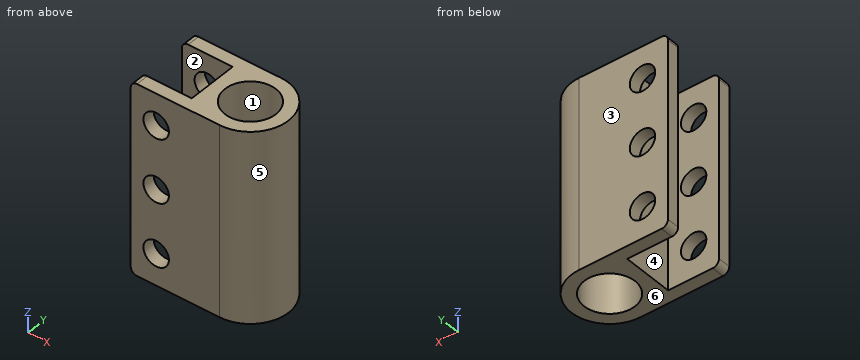
from build123d import *

# Parameters (mm, degrees)
F0_R     = 20
F1_DEPTH = 75
F2_W     = 40
F2_H     = 150
F3_DEPTH = 40
F4_R     = 10
F5_DEPTH = 60
F6_R     = 5
F7_T     = -2


with BuildPart() as f1:
    # F0 (on Top) → F1 (new body, symmetric)
    with BuildSketch(Plane.XY):
        with BuildLine():
            ThreePointArc((30, 0), (21.2132034356, 21.2132034356), (0, 30))
            ThreePointArc((0, 30), (-30, 0), (0, -30))
            ThreePointArc((0, -30), (21.2132034356, -21.2132034356), (30, 0))
        make_face()
        Circle(F0_R, mode=Mode.SUBTRACT)
        with BuildLine():
            Line((0, 30), (-70, 30))
            Line((-70, 30), (-70, -30))
            Line((-70, -30), (0, -30))
            ThreePointArc((0, -30), (-30, 0), (0, 30))
        make_face()
    extrude(amount=F1_DEPTH, both=True)

    # F2 (on face) → F3 (cut)
    with BuildSketch(Plane(origin=(-70, 0, 0), x_dir=(0, -1, 0), z_dir=(-1, 0, 0))):
        Rectangle(F2_W, F2_H)
    extrude(amount=-F3_DEPTH, mode=Mode.SUBTRACT)

    # F4 (on face) → F5 (cut)
    with BuildSketch(Plane.XZ.offset(30)):
        with Locations((-50, 50)):
            Circle(F4_R)
        with Locations((-50, 0)):
            Circle(F4_R)
        with Locations((-50, -50)):
            Circle(F4_R)
    extrude(amount=-F5_DEPTH, mode=Mode.SUBTRACT)

    # F6
    f6_edges = [f1.edges().sort_by_distance(p)[0] for p in [
        (-70, 25, 75),
        (-70, -25, 75),
        (-70, 25, -75),
        (-70, -25, -75),
    ]]
    fillet(f6_edges, radius=F6_R)

    # F7 (hollow: no face is removed)
    offset(amount=F7_T, kind=Kind.INTERSECTION, mode=Mode.SUBTRACT)


solid = f1.part
Geometry check sheet. Reference: the model listing, model coordinates, mm. Face numbers are marked on the shaded views. A direction names the side the tool comes from. Round coordinates to 2 decimals unless told otherwise and drop trailing zeros. Order: outer loops, then holes, each group sorted by start corner. A loop starts at its lowest first (then second) coordinate and runs counter-clockwise, first axis right, second up. Notation, with made-up numbers: M 13.5,25 L 72.5,25 A10 ccw 72.5,44 Z; hole C 13.5,36.25 d10. An arc over 180 degrees is marked long. Answer in a Markdown table with one row per item. Add a question column.
Item 1: Set-up check for the marked faces 1 and 2: record each of +Z, -Z, +X, -X, +Y, -Y from which the full face is reachable in a straight line by a thin tool's end or side.
Item 2: Sectioned sample at C-C, the plane x = 3. Enter the section's corners in (y, z).
Item 3: Sectioned sample at D-D, the plane z = 20. Enter the section's corners in (x, y).
Item 4: Material ranges on L1, parallel to Y at x = -30.5, z = -49.5; L2, parallel to Y at x = -29, z = -47.5; L3, parallel to Y at x = 13, z = -7, recorded low to high. Write a range as [from, to].
Item 5: Draft check along Y on the marked faces 3, 4, 5 and 6. Enter one of: released by +Y, released by -Y, zero draft, split by the parting line, or undercut.
Item 6: Sectioned sample at B-B, the plane z = 50. State how many separate pieces and enclosed holes the cut face has, plus the area to 3 significant figures.
Item 7: Depth check by flat-ended pin: pin 1 Ø12 at (y, z) = (14, 51.5) entering from +X; pin 2 Ø6 at (y, z) = (3, 20) entering from -X; pin 3 Ø12 at (x, z) = (-50, -50) entering from -Y; pin 4 Ø12 at (y, z) = (12, 57.5) entering from +X. Enter the tip coordinate at first touch or a pass-through.
Item 8: Sectioned sample at A-A, the plane y = 0. Enter the section's corners in (x, z).
Filled in:
| question | item | result |
|---|---|---|
| 1 | face 1 | +Z, -Z |
| 1 | face 2 | +Z, -Z, -X |
| 2 | outline | M -29.85,-75 L -19.77,-75 L -19.77,75 L -29.85,75 Z; M 19.77,-75 L 29.85,-75 L 29.85,75 L 19.77,75 Z; hole M -27.84,-73 L -21.79,-73 L -21.79,73 L -27.84,73 Z; hole M 21.79,-73 L 27.84,-73 L 27.84,73 L 21.79,73 Z |
| 3 | outline | M -70,-30 L 0,-30 A30 ccw 0,30 L -70,30 L -70,20 L -30,20 L -30,-20 L -70,-20 Z; C 0,0 d44; hole M -68,-28 L 0,-28 A28 ccw 0,28 L -68,28 L -68,22 L -28,22 L -28,-22 L -68,-22 Z; hole C 0,0 d40 |
| 4 | L1 | y = [-30, -28], [-22, -20], [20, 22], [28, 30] |
| 4 | L2 | y = [-30, -28], [-22, 22], [28, 30] |
| 4 | L3 | y = [-27.04, -24.8], [-17.75, -15.2], [15.2, 17.75], [24.8, 27.04] |
| 5 | face 3 | released by +Y |
| 5 | face 4 | undercut |
| 5 | face 5 | split by the parting line |
| 5 | face 6 | zero draft |
| 6 | separate pieces | 4 |
| 6 | enclosed holes | 4 |
| 6 | area | 886 mm² |
| 7 | pin 1 | stops at x = 28.91 |
| 7 | pin 2 | stops at x = -30 |
| 7 | pin 3 | passes through |
| 7 | pin 4 | stops at x = 29.39 |
| 8 | outline | M -30,-75 L -20,-75 L -20,75 L -30,75 Z; M 20,-75 L 30,-75 L 30,75 L 20,75 Z; hole M -28,-73 L -22,-73 L -22,73 L -28,73 Z; hole M 22,-73 L 28,-73 L 28,73 L 22,73 Z |
